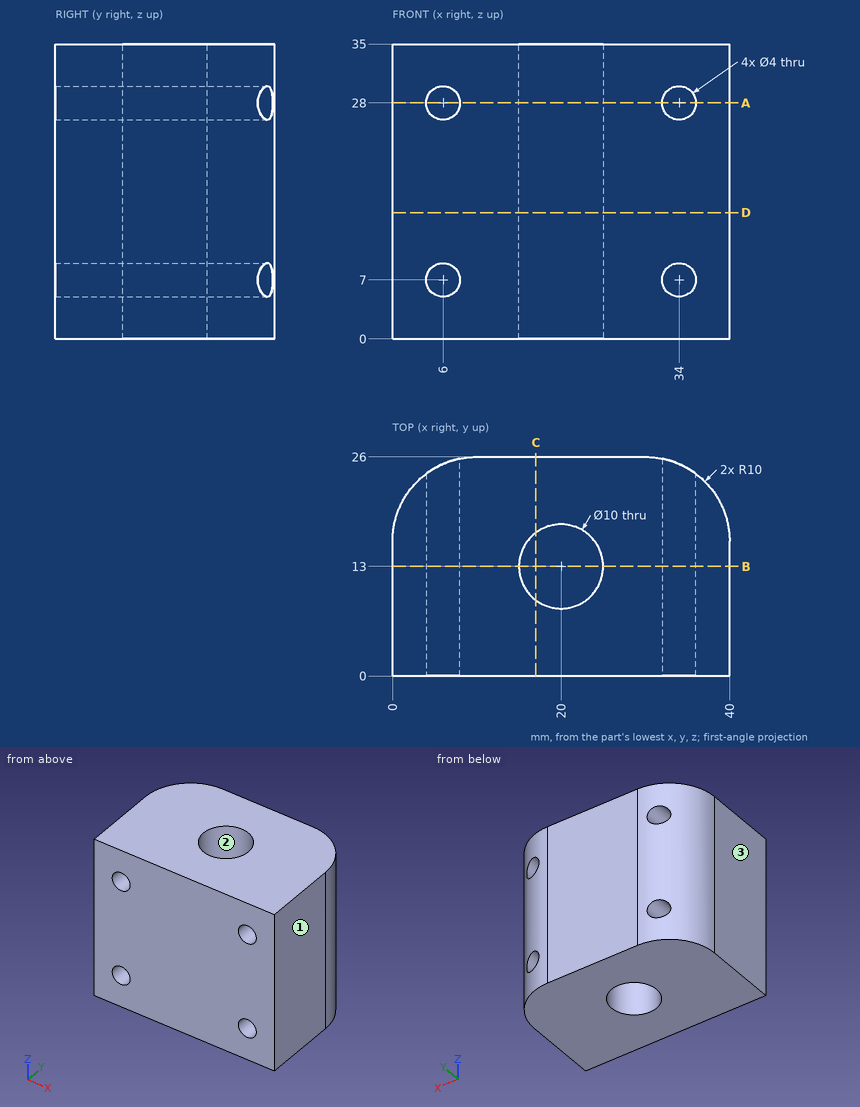
Part print with two shaded views. Sizes in mm from the minimum x, y, z corner. Round coordinates to 2 decimals unless told otherwise and drop trailing zeros. Order: outer loops, then holes, each group sorted by start corner. A loop starts at its lowest first (then second) coordinate and runs counter-clockwise, first axis right, second up. Notation, with made-up numbers: M 64,-36.75 L 109,-36.75 A6 cw 109,-31.75 Z; hole C 74,33 d11. An arc over 180 degrees is marked long. Put each result on its own line as item: value. Start each with the question number.
1. Slice it at C-C on x = 17. List the corners of the cut face in (y, z).
2. Drill centre lines: probe 1 along Z at (x, y) = (34, 14.25); probe 2 along Y at (x, z) = (20, 33); probe 3 along Y at (x, z) = (18, 20). Where is each one in solid material? Low to high. Write a range as [from, to].
3. Slice it at D-D on z = 15. List the corners of the cut face in (x, y), then the cut area to 3 significant figures.
4. Two-plate mould, pull along X, no slides. Class the marked faces 1, 2 and 3: +X half, -X half, draft (parallel to the pull), parting line (faces both ways), or undercut.
5. Slice it at A-A on z = 28. List the corners of the cut face in (x, y).
6. Slice it at B-B on y = 13. List the corners of the cut face in (x, z), then the cut area to 4 significant figures.
Findings:
1. outline: M 0,0 L 9,0 L 9,35 L 0,35 Z; M 17,0 L 26,0 L 26,35 L 17,35 Z
2. probe 1: [0, 5], [9, 26], [30, 35]
2. probe 2: [0, 8], [18, 26]
2. probe 3: [0, 8.42], [17.58, 26]
3. outline: M 0,0 L 40,0 L 40,16 A10 ccw 30,26 L 10,26 A10 ccw 0,16 Z; hole C 20,13 d10
3. area: 919 mm2
4. face 1: +X half
4. face 2: undercut
4. face 3: -X half
5. outline: M 0,0 L 4,0 L 4,24 A10 ccw 0,16 Z; M 8,0 L 32,0 L 32,25.8 A10 ccw 30,26 L 10,26 A10 ccw 8,25.8 Z; M 36,0 L 40,0 L 40,16 A10 ccw 36,24 Z; hole C 20,13 d10
6. outline: M 0,0 L 15,0 L 15,35 L 0,35 Z; M 25,0 L 40,0 L 40,35 L 25,35 Z; hole C 6,7 d4; hole C 6,28 d4; hole C 34,7 d4; hole C 34,28 d4
6. area: 1,000 mm2
